```python
from build123d import *

# Parameters (mm, degrees)
EXTRUDE1_DEPTH = 0.05
EXTRUDE2_DEPTH = 0.9
SKETCH5_W      = 8.3
SKETCH5_H      = 15.2
EXTRUDE3_DEPTH = 5.6


with BuildPart() as part:
    # Sketch1 → Extrude1 (new body)
    with BuildSketch(Plane(origin=(0, 0, 0), x_dir=(1, 0, 0), z_dir=(0, 1, 0))):
        Polygon((0, 0), (0.12, 10), (2.25, 10), (2.25, 42.8), (4.15, 42.8), (4.15, 60), (-4.15, 60), (-4.15, 42.8), (-2.25, 42.8), (-2.25, 10), (-0.12, 10), align=None)
    extrude(amount=EXTRUDE1_DEPTH)

    # Sketch4 → Extrude2 (add)
    with BuildSketch(Plane(origin=(0, 0.05, 0), x_dir=(1, 0, 0), z_dir=(0, 1, 0))):
        Polygon((-4.15, 60), (4.15, 60), (4.15, 42.8), (2.25, 42.8), (2.25, 10), (-2.25, 10), (-2.25, 42.8), (-4.15, 42.8), align=None)
    extrude(amount=EXTRUDE2_DEPTH)

    # Sketch5 → Extrude3 (add)
    with BuildSketch(Plane(origin=(0, 0.95, 0), x_dir=(1, 0, 0), z_dir=(0, 1, 0))):
        with Locations((0, 50.4)):
            Rectangle(SKETCH5_W, SKETCH5_H)
    extrude(amount=EXTRUDE3_DEPTH)


solid = part.part
```
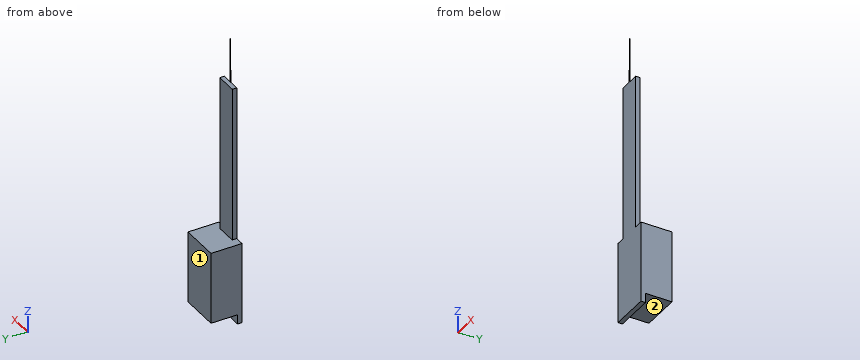
The listing builds one solid part. Answer for the finished solid, in the listing's coordinates (mm). Face numbers are marked on the shaded views. A direction names the side the tool comes from. Round coordinates to 2 decimals unless told otherwise and drop trailing zeros. Loops run counter-clockwise (first coordinate to the right, second up) from the corner with the lowest first, then second, coordinate; pieces in that order, holes last.
Q1. Find the intervals of material crossed by line 1 (Y direction, x = -1.5, z = -40); line 2 (Z direction, x = -0.5, y = 4.75), in increasing order.
Q2. Section C-C, the plane z = -16 is taken. Determine the outline of the cut face in (x, y).
Q3. Which of the six approach directions +Z, -Z, +X, -X, +Y, -Y give full straight-line access (tool end or side, diameter ignored) to the marked faces 1 and 2?
Q4. Section B-B, the plane y = 5.25 is taken. Determine the outline of the cut face in (x, z).
Q5. Section A-A, the plane x = 1.75 is taken. Determine the outline of the cut face in (y, z), then the cut area to 3 significant figures.
Q6. Given pin 1 Ø3 at (x, y) = (-2, 1.5) entering from -Z; pin 2 Ø3 at (x, z) = (-1, -36) entering from +Y; pin 3 Ø0.5 at (x, y) = (0.5, 0.5) entering from +Z; pin 4 Ø0.5 at (y, z) = (0.5, -28) entering from +X, each flat-ended and moving along its own axis, determine where each tip first touches the part or whether it passes through.
Completed:
1. line 1: y = 0 to 0.95
1. line 2: z = -58 to -42.8
2. outline: (-2.25, 0) - (2.25, 0) - (2.25, 0.95) - (-2.25, 0.95) - close
3. face 1: +Z, -Z, +X, -X, +Y
3. face 2: -Z, +X, -X, +Y
4. outline: (-4.15, -58) - (4.15, -58) - (4.15, -42.8) - (-4.15, -42.8) - close
5. outline: (0, -60) - (0.95, -60) - (0.95, -58) - (6.55, -58) - (6.55, -42.8) - (0.95, -42.8) - (0.95, -10) - (0, -10) - close
5. area: 133 mm2
6. pin 1: stops at z = -60
6. pin 2: stops at y = 0.95
6. pin 3: stops at z = -10
6. pin 4: stops at x = 2.25
